Geometry check sheet. Reference: the model listing, model coordinates, mm. Face numbers are marked on the shaded views. A direction names the side the tool comes from. Round coordinates to 2 decimals unless told otherwise and drop trailing zeros. Write each loop counter-clockwise with the first axis right and the second up, starting at its lowest first coordinate (ties: lowest second). Pieces come first, ordered by that corner, then holes.
Item 1: Draft check along Y on the marked faces 1, 2 and 3. Enter one of: pulls with the +Y half, pulls with the -Y half, needs draft (parallel to the pull), parting line crosses it, or undercut.
Item 2: Cross-section at B-B (z = 8). Enter the section's corners in (x, y), then the cut area to 3 significant figures.
Item 3: Scan lines: probe 1 along Y at (x, z) = (0, 68); probe 2 along Z at (x, y) = (-17, 18); probe 3 along Y at (x, z) = (-7, 53) (3 decimals). Record each from-to range of solid material in increasing order.
Item 4: Access from +Z, -Z, +X, -X, +Y, -Y to the whole of each face (thin tool, end or side, straight path). Record for the marked faces 4, 5 and 6.
Item 5: Depth check by flat-ended pin: P1, Ø5, axis at x = 12.84, y = 4.17, coming from the +Z side; P2, Ø1, axis at y = 15.5, z = 58.5, coming from the -X side; P3, Ø10, axis at y = -9, z = 28, coming from the -X side; P4, Ø7, axis at x = -7.94, y = -10.92, coming from the +Z side. Enter the tip coordinate at first touch or a pass-through.
Item 6: Cross-section at A-A (x = 0). State how many separate pieces and enclosed holes the cut face has, then the cut area to 3 significant figures.
from build123d import *

# Parameters (mm, degrees)
SKETCH_1_R          = 10
EXTRUDE_1_DEPTH     = 20
SKETCH_2_R          = 17.5
EXTRUDE_2_DEPTH     = 41
SKETCH_3_R          = 17.5
EXTRUDE_3_DEPTH     = 10
SKETCH_8_R          = 3
CUT_EXTRUDE_4_DEPTH = 60
EXTRUDE_START       = -8
SKETCH_9_R          = 30
SKETCH_9_R_2        = 17.5
EXTRUDE_4_DEPTH     = 8
EXTRUDE_START_2     = 17
SKETCH_10_R         = 20
SKETCH_10_R_2       = 17.5
EXTRUDE_5_DEPTH     = 17
CHAMFER_1_SIZE      = 0.5
CHAMFER_2_SIZE      = 0.5
SKETCH_12_R         = 5.5
CUT_EXTRUDE_6_DEPTH = 6
SKETCH_13_R         = 3
CUT_EXTRUDE_7_DEPTH = 8


with BuildPart() as part:
    # 草图1 → 拉伸1 (new body)
    with BuildSketch(Plane.XY):
        Circle(SKETCH_1_R)
    extrude(amount=EXTRUDE_1_DEPTH)

    # 草图2 → 拉伸2 (add)
    with BuildSketch(Plane.XY.offset(20)):
        Circle(SKETCH_2_R)
    extrude(amount=EXTRUDE_2_DEPTH)

    # 草图3 → 拉伸3 (add)
    with BuildSketch(Plane.XY.offset(61)):
        Circle(SKETCH_3_R)
    extrude(amount=EXTRUDE_3_DEPTH)

    # 草图8 → 切除-拉伸4 (cut)
    with BuildSketch(Plane.XY.offset(71)):
        with Locations((12.83926297, 4.171729424)):
            Circle(SKETCH_8_R)
        with Locations((0, 13.5)):
            Circle(SKETCH_8_R)
        with Locations((7.935100906, -10.921729424)):
            Circle(SKETCH_8_R)
        with Locations((-7.935100906, -10.921729424)):
            Circle(SKETCH_8_R)
        with Locations((-12.83926297, 4.171729424)):
            Circle(SKETCH_8_R)
    extrude(amount=-CUT_EXTRUDE_4_DEPTH, mode=Mode.SUBTRACT)

    # 草图9 → 拉伸4 (add)
    with BuildSketch(Plane.XY.offset(71).offset(EXTRUDE_START)):
        Circle(SKETCH_9_R)
        Circle(SKETCH_9_R_2, mode=Mode.SUBTRACT)
    extrude(amount=EXTRUDE_4_DEPTH)

    # 草图10 → 拉伸5 (add)
    with BuildSketch(Plane(origin=(0, 0, 63), x_dir=(-1, 0, 0), z_dir=(0, 0, -1)).offset(EXTRUDE_START_2)):
        with Locations(Location((0, 0, 0), (0, 0, 180))):
            Circle(SKETCH_10_R)
        Circle(SKETCH_10_R_2, mode=Mode.SUBTRACT)
    extrude(amount=-EXTRUDE_5_DEPTH)

    # 倒角1
    chamfer_1_edges = [part.edges().sort_by_distance(p)[0] for p in [
        (-17.5, 0, 20),
    ]]
    chamfer(chamfer_1_edges, length=CHAMFER_1_SIZE)

    # 倒角2
    chamfer_2_edges = [part.edges().sort_by_distance(p)[0] for p in [
        (-10, 0, 0),
        (-30, 0, 63),
        (-30, 0, 71),
        (-20, 0, 46),
    ]]
    chamfer(chamfer_2_edges, length=CHAMFER_2_SIZE)

    # 草图12 → 切除-拉伸6 (cut)
    with BuildSketch(Plane.XY.offset(71)):
        with Locations((0, 13.5)):
            Circle(SKETCH_12_R)
        with Locations((12.83926297, 4.171729424)):
            Circle(SKETCH_12_R)
        with Locations((7.935100906, -10.921729424)):
            Circle(SKETCH_12_R)
        with Locations((-7.935100906, -10.921729424)):
            Circle(SKETCH_12_R)
        with Locations((-12.83926297, 4.171729424)):
            Circle(SKETCH_12_R)
    extrude(amount=-CUT_EXTRUDE_6_DEPTH, mode=Mode.SUBTRACT)

    # 草图13 → 切除-拉伸7 (cut)
    with BuildSketch(Plane.XY.offset(71)):
        with Locations((0, 25)):
            Circle(SKETCH_13_R)
        with Locations((21.650635095, 12.5)):
            Circle(SKETCH_13_R)
        with Locations((21.650635095, -12.5)):
            Circle(SKETCH_13_R)
        with Locations((0, -25)):
            Circle(SKETCH_13_R)
        with Locations((-21.650635095, -12.5)):
            Circle(SKETCH_13_R)
        with Locations((-21.650635095, 12.5)):
            Circle(SKETCH_13_R)
    extrude(amount=-CUT_EXTRUDE_7_DEPTH, mode=Mode.SUBTRACT)


solid = part.part
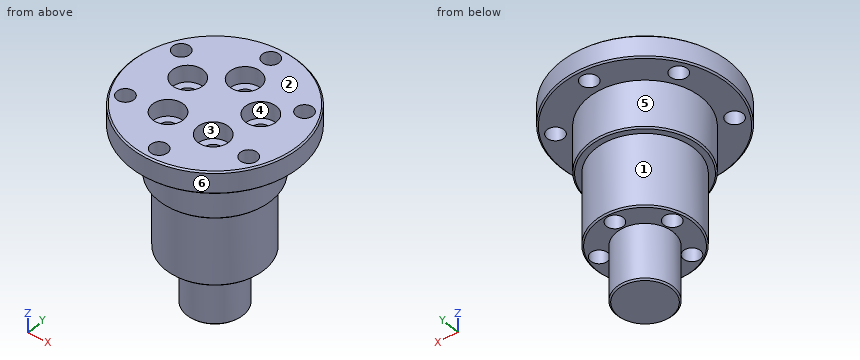
Resolved:
1. face 1: parting line crosses it
1. face 2: needs draft
1. face 3: undercut
2. outline: circle Ø20 at (0, 0)
2. area: 314 mm2
3. probe 1: y = -30 to -28, -22 to 8, 19 to 22, 28 to 30
3. probe 2: z = 63 to 71
3. probe 3: y = -18.735 to -13.772, -8.071 to 18.735
4. face 4: +Z
4. face 5: -Z
4. face 6: +Z, -Z
5. P1: passes through
5. P2: stops at x = -13.23
5. P3: stops at x = -17.04
5. P4: stops at z = 65
6. separate pieces: 4
6. enclosed holes: 0
6. area: 2,040 mm2
